from build123d import *

# Parameters (mm, degrees)
SKETCH1_W           = 256
SKETCH1_H           = 248.2
BOSS_EXTRUDE1_DEPTH = 2
SKETCH2_W           = 256
SKETCH2_H           = 2
BOSS_EXTRUDE2_DEPTH = 4
SKETCH3_W           = 256
SKETCH3_H           = 1.999419648
BOSS_EXTRUDE3_DEPTH = 1.89
SKETCH4_W           = 256
SKETCH4_H           = 2
BOSS_EXTRUDE4_DEPTH = 1.89
SKETCH5_W           = 33.5
SKETCH5_H           = 3.89
CUT_EXTRUDE1_DEPTH  = 10
BOSS_EXTRUDE5_DEPTH = 20


with BuildPart() as part:
    # Sketch1 → Boss-Extrude1 (new body)
    with BuildSketch(Plane(origin=(0, 0, 0), x_dir=(1, 0, 0), z_dir=(0, 1, 0))):
        Rectangle(SKETCH1_W, SKETCH1_H)
    extrude(amount=BOSS_EXTRUDE1_DEPTH)

    # Sketch2 → Boss-Extrude2 (add)
    with BuildSketch(Plane(origin=(0, 2, 0), x_dir=(1, 0, 0), z_dir=(0, 1, 0))):
        with Locations((0, -123.1)):
            Rectangle(SKETCH2_W, SKETCH2_H)
        with Locations((0, 123.1)):
            Rectangle(SKETCH2_W, SKETCH2_H)
    extrude(amount=BOSS_EXTRUDE2_DEPTH)

    # Sketch3 → Boss-Extrude3 (add)
    with BuildSketch(Plane(origin=(0, 0, 122.1), x_dir=(-1, 0, 0), z_dir=(0, 0, -1))):
        with Locations((0, 5.000290176)):
            Rectangle(SKETCH3_W, SKETCH3_H)
    extrude(amount=BOSS_EXTRUDE3_DEPTH)

    # Sketch4 → Boss-Extrude4 (add)
    with BuildSketch(Plane.XY.offset(-122.1)):
        with Locations((0, 5)):
            Rectangle(SKETCH4_W, SKETCH4_H)
    extrude(amount=BOSS_EXTRUDE4_DEPTH)

    # Sketch5 → Cut-Extrude1 (cut)
    with BuildSketch(Plane(origin=(0, 2, 0), x_dir=(1, 0, 0), z_dir=(0, 1, 0))):
        with Locations((111.25, -122.155)):
            Rectangle(SKETCH5_W, SKETCH5_H)
        with Locations((111.25, 122.155)):
            Rectangle(SKETCH5_W, SKETCH5_H)
    extrude(amount=CUT_EXTRUDE1_DEPTH, mode=Mode.SUBTRACT)

    # Sketch6 → Boss-Extrude5 (add)
    with BuildSketch(Plane(origin=(0, 2, 0), x_dir=(1, 0, 0), z_dir=(0, 1, 0))):
        Polygon((94.5, -124.1), (94.5, -122.1), (126, -122.1), (126, 122.1), (94.5, 122.1), (94.5, 124.1), (128, 124.1), (128, -124.1), align=None)
    extrude(amount=BOSS_EXTRUDE5_DEPTH)


solid = part.part
Input: part model. Units: mm. Frame: model coordinates. Round coordinates to 2 decimals unless told otherwise and drop trailing zeros. Order: outer loops, then holes, each group sorted by start corner. A loop starts at its lowest first (then second) coordinate and runs counter-clockwise, first axis right, second up.
1. Material intervals for line 1 (Z direction, x = 111, y = 3); line 2 (Z direction, x = -115, y = 4.75); line 3 (Y direction, x = 4, z = -86.5), sorted ascending.
The answers:
line 1: z = -124.1 to -122.1, 122.1 to 124.1
line 2: z = -124.1 to -120.21, 120.21 to 124.1
line 3: y = 0 to 2
2. Cut plane B-B, the plane x = 47. Output: boundary loops of the cut face in (y, z).
The answers:
outline: (0, -124.1) - (6, -124.1) - (6, -120.21) - (4, -120.21) - (4, -122.1) - (2, -122.1) - (2, 122.1) - (4, 122.1) - (4, 120.21) - (6, 120.21) - (6, 124.1) - (0, 124.1) - close
3. Pin query (flat end, axial travel): P1, Ø1, axis at x = 89, z = -33, coming from the +Y side; P2, Ø0.6, axis at y = 14.5, z = -123, coming from the -X side; P3, Ø1.2, axis at x = 36, z = -122, coming from the +Y side; P4, Ø12, axis at x = 82.5, y = 14, coming from the -Z side. Return the tip coordinate at first contact, or that it passes through.
The answers:
P1: stops at y = 2
P2: stops at x = 94.5
P3: stops at y = 6
P4: passes through
4. Cut plane A-A, the plane y = 14. Output: boundary loops of the cut face in (x, z).
The answers:
outline: (94.5, -124.1) - (128, -124.1) - (128, 124.1) - (94.5, 124.1) - (94.5, 122.1) - (126, 122.1) - (126, -122.1) - (94.5, -122.1) - close
5. Cut plane C-C, the plane z = -40.5. Output: boundary loops of the cut face in (x, y).
The answers:
outline: (-128, 0) - (128, 0) - (128, 22) - (126, 22) - (126, 2) - (-128, 2) - close
